Geometry check sheet. Reference: the model listing, model coordinates, mm. A direction names the side the tool comes from. Coordinates: 2 decimals unless noted, no trailing zeros. Write each loop counter-clockwise with the first axis right and the second up, starting at its lowest first coordinate (ties: lowest second). Pieces come first, ordered by that corner, then holes. Notation, with made-up numbers: M 84,39 L 120,39 A7 ccw 120,48 Z; hole C 74.5,-17.5 d3. An arc over 180 degrees is marked long. Write each question's results on one line, items separated by ' | '.
```python
from build123d import *

# Parameters (mm, degrees)
F0_W     = 558.8
F0_H     = 736.6
F1_DEPTH = 381
F3_DEPTH = 279.4
F5_DEPTH = 101.6
F6_R     = 50.8
F7_R     = 76.2


with BuildPart() as f1:
    # F0 (on Top) → F1 (new body)
    with BuildSketch(Plane.XY):
        Rectangle(F0_W, F0_H)
    extrude(amount=F1_DEPTH)

    # F2 (on Right) → F3 (join, symmetric)
    with BuildSketch(Plane.YZ):
        Polygon((-1631.65164, 381), (-368.3, 190.5), (-368.3, 381), (-1631.65164, 571.754465), align=None)
    extrude(amount=F3_DEPTH, both=True)

    # F4 (on Right) → F5 (join, symmetric)
    with BuildSketch(Plane.YZ):
        with BuildLine():
            Line((-1877.153158, 518.437564), (-1631.65164, 449.142784))
            Line((-1631.65164, 449.142784), (-1631.65164, 526.356995))
            Line((-1631.65164, 526.356995), (-1679.167986, 548.13534))
            ThreePointArc((-1679.167986, 548.13534), (-1806.758775, 608.180538), (-1944.468141, 577.833116))
            Line((-1944.468141, 577.833116), (-1877.153158, 518.437564))
        make_face()
    extrude(amount=F5_DEPTH, both=True)

    # F6
    f6_edges = [f1.edges().sort_by_distance(p)[0] for p in [
        (279.4, -999.97582, 476.377233),
        (-279.4, -999.97582, 476.377233),
        (-279.4, -1631.65164, 476.377233),
        (279.4, -1631.65164, 476.377233),
    ]]
    fillet(f6_edges, radius=F6_R)

    # F7
    f7_edges = [f1.edges().sort_by_distance(p)[0] for p in [
        (0, 368.3, 381),
    ]]
    fillet(f7_edges, radius=F7_R)


solid = f1.part
```
Q1. Sectioned sample at B-B on y = 148.5. Record the cut outline in (x, z).
Geometry check:
outline: M -279.4,0 L 279.4,0 L 279.4,381 L -279.4,381 Z
Q2. Sectioned sample at A-A on x = 183.5. Record the cut outline in (y, z).
Geometry check:
outline: M -1631.65,381 L -368.3,190.5 L -368.3,0 L 368.3,0 L 368.3,304.8 A76.2 ccw 292.1,381 L -368.3,381 L -1631.65,571.75 Z
Q3. Mould release check, pull along Y, two halves, no side actions. Record for faces 6 (the flat face through (1.422, -1756.121, 484.275)), 7 (the flat face through (3, -1631.652, 435)), 8 (the flat face through (3.2, -991.13, 475.04)): pulls with the +Y half, pulls with the -Y half, needs draft (parallel to the pull), parting line crosses it, or undercut.
Geometry check:
face 6: pulls with the -Y half | face 7: undercut | face 8: pulls with the +Y half
Q4. Depth check by flat-ended pin: P1, Ø10, axis at x = 41.5, z = 145, coming from the -Y side; P2, Ø12, axis at x = -51.5, y = -735, coming from the +Z side; P3, Ø2, axis at x = -204.5, z = 501, coming from the -Y side. Enter the tip coordinate at first touch or a pass-through.
Geometry check:
P1: stops at y = -368.3 | P2: stops at z = 437.27 | P3: stops at y = -1631.65
Q5. Access from +Z, -Z, +X, -X, +Y, -Y to the whole of each face (thin tool, end or side, straight path). Record for faces 1 (the flat face through (-279.4, -403, 260)), 2 (the flat face through (279.4, -403, 260)), 3 (the flat face through (-4, -368.3, 94)), 4 (the flat face through (-101.6, -1790, 530)), 5 (the flat face through (101.6, -1790, 530)).
Geometry check:
face 1: +Z, -Z, -X, +Y, -Y | face 2: +Z, -Z, +X, +Y, -Y | face 3: -Z, +X, -X, -Y | face 4: +Z, -Z, -X, -Y | face 5: +Z, -Z, +X, -Y
Q6. Sectioned sample at C-C on z = 165. Record the cut outline in (x, y).
Geometry check:
outline: M -279.4,-368.3 L 279.4,-368.3 L 279.4,368.3 L -279.4,368.3 Z
Q7. Sectioned sample at D-D on x = -76. Record the cut outline in (y, z).
Geometry check:
outline: M -1944.47,577.83 L -1877.15,518.44 L -1631.65,449.14 L -1631.65,381 L -368.3,190.5 L -368.3,0 L 368.3,0 L 368.3,304.8 A76.2 ccw 292.1,381 L -368.3,381 L -1631.65,571.75 L -1631.65,526.36 L -1679.17,548.14 A218.62 ccw Z
Q8. Scan lines: probe 1 along Z at (x, y) = (-239, -73); probe 2 along Y at (x, z) = (190, 184); probe 3 along X at (y, z) = (-1805, 527). Record each from-to range of solid material in increasing order.
Geometry check:
probe 1: z = 0 to 381 | probe 2: y = -368.3 to 368.3 | probe 3: x = -101.6 to 101.6
